For this review, take the finished solid that the model builds, in its own axes (mm). Face numbers are marked on the shaded views. A direction names the side the tool comes from. Round coordinates to 2 decimals unless told otherwise and drop trailing zeros. Write each loop counter-clockwise with the first axis right and the second up, starting at its lowest first coordinate (ties: lowest second). Pieces come first, ordered by that corner, then holes. Notation, with made-up numbers: (84, 13) -> (88, 13) arc R18 cw to (88, 30) -> close; hole circle Ø1 at (44, 16). An arc over 180 degrees is marked (long way). Write each question's results on one line, items separated by ' | '. Start each with the question number.
Item 1: Add section B-B (y = 7). State the section outline as (x, z) points, plus the area to 3 significant figures.
Item 2: The part is to be moulded in two halves that separate along Y. For the marked faces 1, 2 and 3, say which applies: +Y half, -Y half, draft (parallel to the pull), parting line (faces both ways), or undercut.
Item 3: Add section C-C (z = -83). State the section outline as (x, y) points, plus the area to 3 significant figures.
Item 4: Clearance check with flat-ended pins moving along their axes: pin 1 (1.5 mm diameter, centred on x = -29, y = -6.5, fed in from -Z); pin 2 (4 mm diameter, centred on x = 21.5, y = 28, fed in from -Z); pin 3 (3 mm diameter, centred on y = -31, z = -26.5, fed in from +X). State where each tip first meets the part, or that it passes through.
Item 5: Add section A-A (x = 0). State the section outline as (y, z) points, plus the area to 3 significant figures.
Item 6: To check wall thickness, follow line 1 along X through (y, z) = (0, -51); line 2 along Y through (x, z) = (0.5, -26). State the ranges of each line that lie inside material, in increasing order.
Item 7: Tool access review of the marked faces 4, 5 and 6: name each direction out of +Z, -Z, +X, -X, +Y, -Y from which nothing blocks a thin tool from reaching the whole face with its end or side.
Item 8: Add section D-D (z = -133.5). State the section outline as (x, y) points.
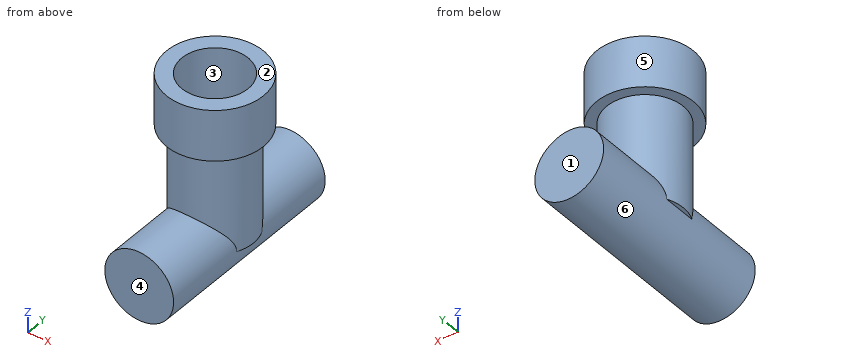
from build123d import *

# Parameters (mm, degrees)
SKETCH_1_R           = 30
SKETCH_1_R_2         = 26
EXTRUDE_1_DEPTH      = 120
SKETCH_2_R           = 38
SKETCH_2_R_2         = 30
EXTRUDE_2_DEPTH      = 40
EXTRUDE_3_DEPTH      = 78
EXTRUDE_3_DEPTH_BACK = 78
SKETCH_3_R           = 27


with BuildPart() as part:
    # Sketch 1 → Extrude 1 (new body)
    with BuildSketch(Plane.XY):
        Circle(SKETCH_1_R)
        Circle(SKETCH_1_R_2, mode=Mode.SUBTRACT)
    extrude(amount=-EXTRUDE_1_DEPTH)

    # Sketch 2 → Extrude 2 (add)
    with BuildSketch(Plane.XY):
        Circle(SKETCH_2_R)
        Circle(SKETCH_2_R_2, mode=Mode.SUBTRACT)
    extrude(amount=-EXTRUDE_2_DEPTH)

    # Sketch 3 → Extrude 3 (add, two sides: drawn at the far end of the back side and taken through both)
    with BuildSketch(Plane(origin=(0, 0, 0), x_dir=(1, 0, 0), z_dir=(0, 1, 0)).offset(-EXTRUDE_3_DEPTH_BACK)):
        with Locations(Location((0, 120, 0), (0, 0, 270))):
            Circle(SKETCH_3_R)
    extrude(amount=EXTRUDE_3_DEPTH + EXTRUDE_3_DEPTH_BACK)


solid = part.part
Responses:
1) outline: (-37.35, -40) -> (-29.17, -40) -> (-29.17, -120) -> (-27, -120) arc R27 ccw to (27, -120) -> (29.17, -120) -> (29.17, -40) -> (37.35, -40) -> (37.35, 0) -> (25.04, 0) -> (25.04, -109.9) arc R27 ccw to (-25.04, -109.9) -> (-25.04, 0) -> (-37.35, 0) -> close | area: 3,910 mm^2
2) face 1: +Y half | face 2: draft | face 3: undercut
3) outline: circle Ø60 at (0, 0); hole circle Ø52 at (0, 0) | area: 704 mm^2
4) pin 1: stops at z = -120 | pin 2: stops at z = -138.67 | pin 3: stops at x = 23.95
5) outline: (-78, -147) -> (78, -147) -> (78, -93) -> (30, -93) -> (30, -40) -> (38, -40) -> (38, 0) -> (26, 0) -> (26, -93) -> (-26, -93) -> (-26, 0) -> (-38, 0) -> (-38, -40) -> (-30, -40) -> (-30, -93) -> (-78, -93) -> close | area: 9,810 mm^2
6) line 1: x = -30 to -26, 26 to 30 | line 2: y = -38 to -26, 26 to 38
7) face 4: +Z, -Z, +X, -X, -Y | face 5: +Z | face 6: none
8) outline: (-23.38, -78) -> (23.38, -78) -> (23.38, 78) -> (-23.38, 78) -> close
